Drawing for the job (mm, zero at the part's lowest x, y, z). Give positions to 0.01 mm unless a question says otherwise; leave off trailing zeros. Order: outer loops, then holes, each group sorted by start corner. A loop starts at its lowest first (then second) coordinate and runs counter-clockwise, first axis right, second up. Notation, with made-up numbers: (81, 20) - (103, 20) arc R19 cw to (103, 32) - close; hole circle Ø4 at (-7, 57.25). An arc over 180 degrees is marked (long way). Use a Markdown table: item, result. Add a question column.
(1) Wall check: line 1 (Y direction, x = 4.25, z = 12.25) (1 decimal); line 2 (Y direction, x = 4, z = 13.5) (1 decimal); line 3 (Z direction, x = 1.5, y = 12). Give the ranges that are in metal, low to high.
(2) Flat gauge pin, fed straight in: pin 1 (10 mm diameter, centred on y = 254.08, z = 9.78, fed in from +X). Where does the tip first touch, or does it go through?
(3) Slice it at B-B (z = 13.75). Write the cut outline in (x, y).
(4) Slice it at A-A (x = 2.5). Write the cut outline in (y, z), then the cut area to 4 significant figures.
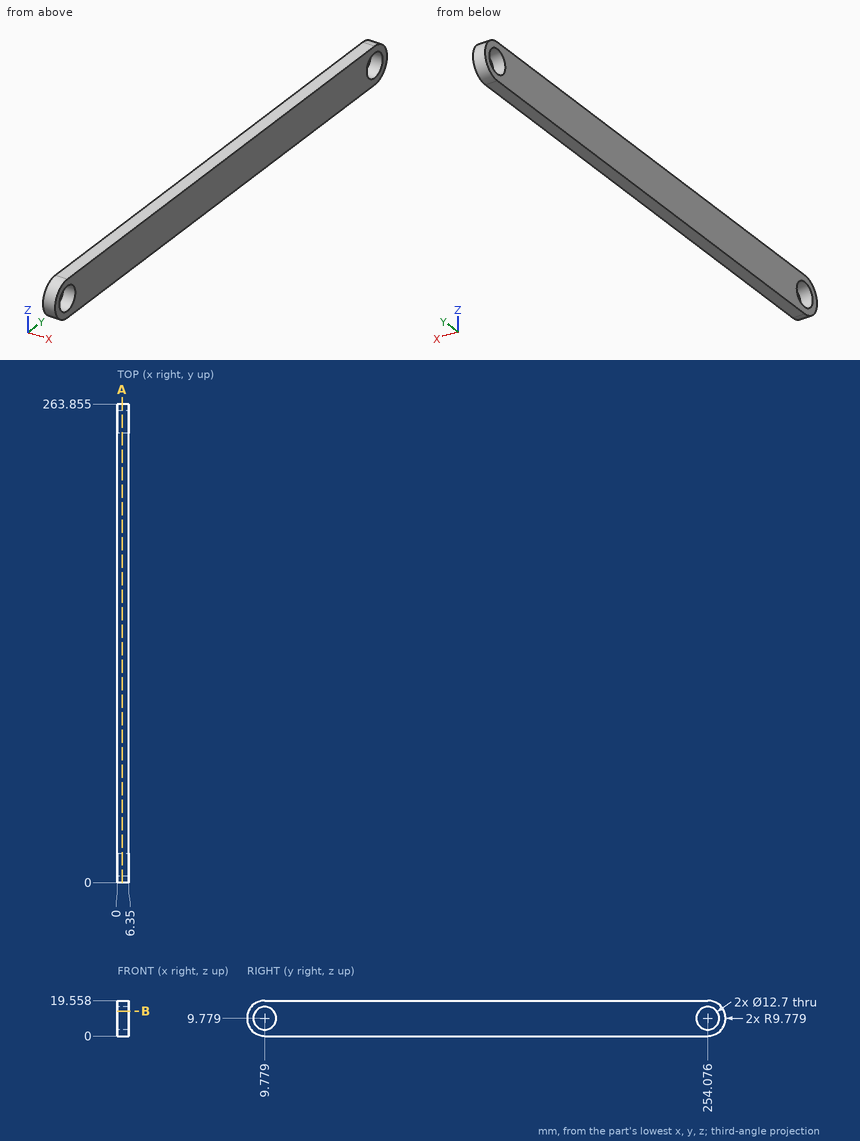
Solution:
| question | item | result |
|---|---|---|
| 1 | line 1 | 0.3 to 3.9, 15.6 to 248.2, 259.9 to 263.5 |
| 1 | line 2 | 0.7 to 4.6, 14.9 to 248.9, 259.2 to 263.1 |
| 1 | line 3 | 0 to 3.83, 15.73 to 19.56 |
| 2 | pin 1 | through |
| 3 | outline | (0, 0.84) - (6.35, 0.84) - (6.35, 4.82) - (0, 4.82) - close; (0, 14.73) - (6.35, 14.73) - (6.35, 249.12) - (0, 249.12) - close; (0, 259.03) - (6.35, 259.03) - (6.35, 263.01) - (0, 263.01) - close |
| 4 | outline | (9.78, 0) - (254.08, 0) arc R9.78 ccw to (254.08, 19.56) - (9.78, 19.56) arc R9.78 ccw to start; hole circle Ø12.7 at (9.78, 9.78); hole circle Ø12.7 at (254.08, 9.78) |
| 4 | area | 4,825 mm2 |
